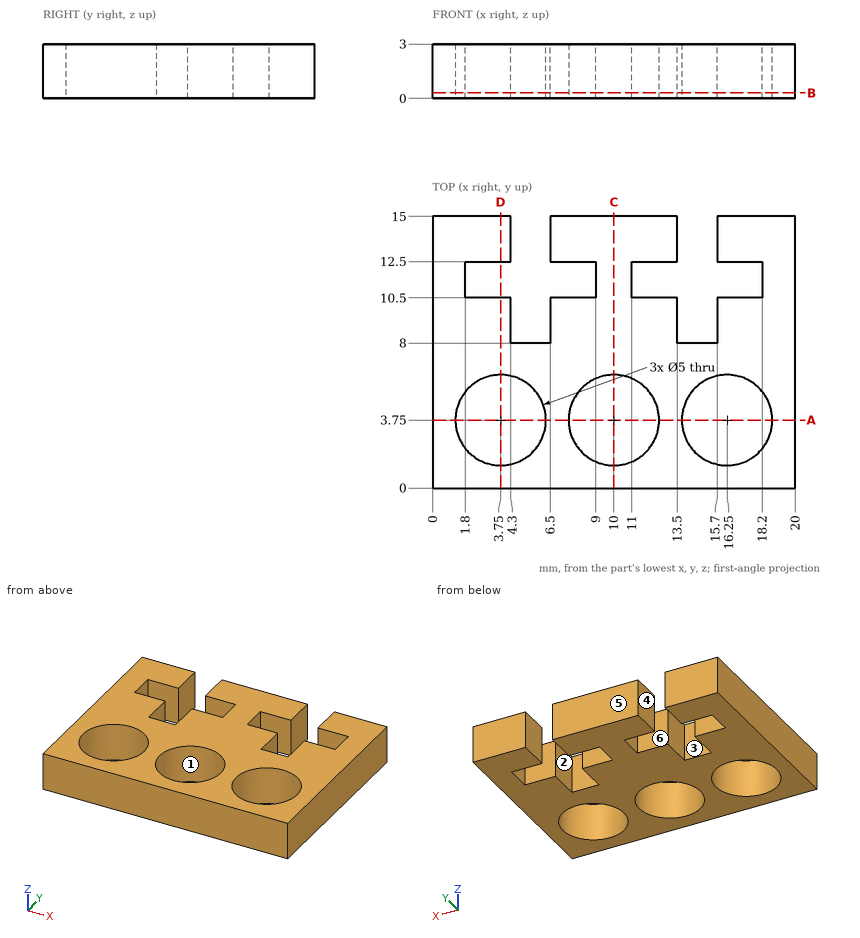
Drawing for the job (mm, zero at the part's lowest x, y, z). A direction names the side the tool comes from. Give positions to 0.01 mm unless a question says otherwise; leave off trailing zeros. Order: outer loops, then holes, each group sorted by start corner. A loop starts at its lowest first (then second) coordinate and runs counter-clockwise, first axis right, second up. Notation, with made-up numbers: M 30.25,64 L 78.25,64 A17 cw 78.25,85 Z; hole C 74,48.5 d3. An arc over 180 degrees is marked long. Put each result on its own line as item: value.
Item 1: 3-axis set-ups, long thin cutter, end or side, ignore diameter. For the marked faces 4, 5 and 6: which of +Z, -Z, +X, -X, +Y, -Y reach the whole face in a straight line?
From the geometry:
face 4: +Z, -Z, +Y
face 5: +Z, -Z, +X, -X, +Y
face 6: +Z, -Z
Item 2: Flat gauge pins, fed straight in: pin 1 Ø6 at (x, y) = (14.5, 4) entering from -Z; pin 2 Ø4.5 at (x, y) = (10, 3.75) entering from -Z. Where does each tip first touch, or does it go through?
From the geometry:
pin 1: stops at z = 0
pin 2: passes through
Item 3: Two-plate mould, pull along Y, no slides. Class the marked faces 1, 2 and 3: +Y half, -Y half, draft (parallel to the pull), parting line (faces both ways), or undercut.
From the geometry:
face 1: undercut
face 2: draft
face 3: +Y half
Item 4: Slice it at B-B, the plane z = 0.3. Give the number of separate pieces and of enclosed holes in the cut face, plus the area to 3 significant figures.
From the geometry:
separate pieces: 1
enclosed holes: 3
area: 190 mm2
Item 5: Slice it at D-D, the plane x = 3.75. Write the cut outline in (y, z).
From the geometry:
outline: M 0,0 L 1.25,0 L 1.25,3 L 0,3 Z; M 6.25,0 L 10.5,0 L 10.5,3 L 6.25,3 Z; M 12.5,0 L 15,0 L 15,3 L 12.5,3 Z
Item 6: Slice it at C-C, the plane x = 10. Write the cut outline in (y, z).
From the geometry:
outline: M 0,0 L 1.25,0 L 1.25,3 L 0,3 Z; M 6.25,0 L 15,0 L 15,3 L 6.25,3 Z
Item 7: Slice it at A-A, the plane y = 3.75. Write the cut outline in (x, z).
From the geometry:
outline: M 0,0 L 1.25,0 L 1.25,3 L 0,3 Z; M 6.25,0 L 7.5,0 L 7.5,3 L 6.25,3 Z; M 12.5,0 L 13.75,0 L 13.75,3 L 12.5,3 Z; M 18.75,0 L 20,0 L 20,3 L 18.75,3 Z
Item 8: Probe line 1 (Y direction, x = 3.75, z = 2.05); line 2 (X direction, y = 12.75, z = 0.25); line 3 (X direction, y = 12, z = 1.8). List the from-to ranges inside material, lowest first. Write a range as [from, to].
From the geometry:
line 1: y = [0, 1.25], [6.25, 10.5], [12.5, 15]
line 2: x = [0, 4.3], [6.5, 13.5], [15.7, 20]
line 3: x = [0, 1.8], [9, 11], [18.2, 20]
